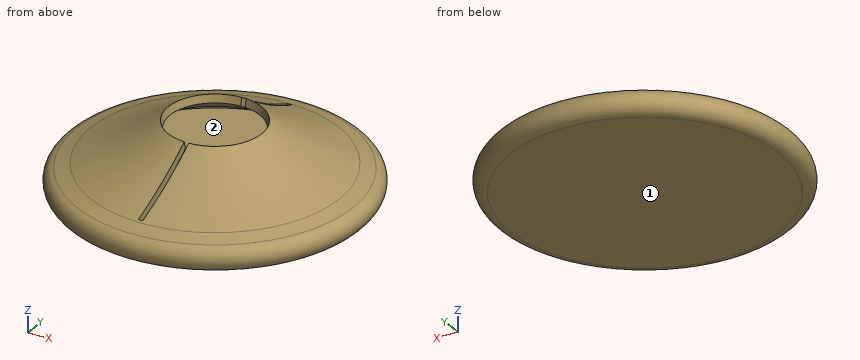
from build123d import *

# Parameters (mm, degrees)
F3_R     = 25
F5_START = -2.7
F4_W     = 1
F4_H     = 53.9998769996
F5_DEPTH = 22.3


# Not quite as in the source:
# - a fillet or chamfer that OpenCascade refuses, or shapes differently, is made with other operations: its cross-section is extruded or revolved along the edge and cut away or added


with BuildPart() as f1:
    # F0 (on Front) → F1 (revolve)
    with BuildSketch(Plane.XZ):
        with BuildLine():
            ThreePointArc((3, 1), (12.6231681205, -4.9677750086), (23, -9.5))
            Line((23, -9.5), (23, -11))
            Line((23, -11), (-7, -11))
            Line((-7, -11), (-7, -13))
            Line((-7, -13), (23, -13))
            ThreePointArc((23, -13), (25.75, -10.25), (23, -7.5))
            ThreePointArc((23, -7.5), (12.6231681205, -2.9677750086), (3, 3))
            Line((3, 3), (3, 1))
        make_face()
    revolve(axis=Axis((-7, 0, -1.698827371), (0, 0, -1)))

    # F2: chamfer of 0.5 x 2 on 1 edges, made by hand

    # F2_s1 → F2_t2 (revolve, cut)
    with BuildSketch(Plane.XZ):
        with BuildLine():
            Line((3.4123952329, 2.7941574241), (2.9820609835, 0.9239297508))
            Line((2.9820609835, 0.9239297508), (2.9420609835, 0.9239297508))
            ThreePointArc((2.9420609835, 0.9239297508), (2.96, 1.9619648754), (2.96, 3))
            Line((2.96, 3), (3.0234608243, 3.0323973722))
            ThreePointArc((3.0234608243, 3.0323973722), (3.2078025867, 2.8993085114), (3.4356565384, 2.8266983471))
            Line((3.4356565384, 2.8266983471), (3.4123952329, 2.7941574241))
        make_face()
    revolve(axis=Axis((-7, 0, 3), (0, 0, -1)), mode=Mode.SUBTRACT)

    # F3
    f3_edges = [f1.edges().sort_by_distance(p)[0] for p in [
        (-37, 0, -7.5),
    ]]
    fillet(f3_edges, radius=F3_R)

    # F4 (on face) → F5 (cut)
    with BuildSketch(Plane(origin=(0, 0, -13), x_dir=(1, 0, 0), z_dir=(0, 0, -1)).offset(F5_START)):
        with Locations((-6.9392545743, 0)):
            Rectangle(F4_W, F4_H)
    extrude(amount=-F5_DEPTH, mode=Mode.SUBTRACT)


solid = f1.part
Input: part model. Units: mm. Frame: model coordinates. Face numbers are marked on the shaded views. Coordinates: 2 decimals unless noted, no trailing zeros.
Q1. Contact query for flat-ended pins moving along their axis: pin 1 (1 mm diameter, centred on x = 0.5, z = -2, fed in from +Y); pin 2 (0.8 mm diameter, centred on x = -7, z = -7.5, fed in from -Y); pin 3 (10 mm diameter, centred on x = 7.5, y = 18.5, fed in from +Z). Output: stop coordinate, or through.
Q2. Material intervals for line 1 (X direction, y = 0, z = -10.4); line 2 (Y direction, x = -7, z = -10.25); line 3 (X direction, y = -1, z = -8), sorted ascending.
Q3. Draft query along Y for the marked faces 1 and 2. Return one class per face: +Y half, -Y half, draft (parallel to the pull), parting line (faces both ways), or undercut.
Working result:
1. pin 1: stops at y = 17.2
1. pin 2: stops at y = -31.43
1. pin 3: stops at z = -2.37
2. line 1: x = -39.75 to -37, 23 to 25.75
2. line 2: y = -32.75 to -30, 30 to 32.75
2. line 3: x = -38.57 to -33.07, 19.07 to 24.57
3. face 1: draft
3. face 2: undercut
